```python
from build123d import *

# Parameters (mm, degrees)
BOSS_EXTRUDE1_DEPTH = 90
BOSS_EXTRUDE2_DEPTH = 38


with BuildPart() as part:
    # Sketch1 → Boss-Extrude1 (new body)
    with BuildSketch(Plane.XY):
        with BuildLine():
            Line((-5, -16.770509831), (-5, -12.8))
            Line((-5, -12.8), (5, -12.8))
            Line((5, -12.8), (5, -16.770509831))
            ThreePointArc((5, -16.770509831), (0, 17.5), (-5, -16.770509831))
        make_face()
    extrude(amount=BOSS_EXTRUDE1_DEPTH)

    # Sketch2 → Boss-Extrude2 (add)
    with BuildSketch(Plane(origin=(0, 0, 0), x_dir=(-1, 0, 0), z_dir=(0, 0, -1))):
        with BuildLine():
            ThreePointArc((-5, -16.770509831), (0, -17.5), (5, -16.770509831))
            Line((5, -16.770509831), (5, -12.8))
            Line((5, -12.8), (-5, -12.8))
            Line((-5, -12.8), (-5, -16.770509831))
        make_face()
    extrude(amount=-BOSS_EXTRUDE2_DEPTH)


solid = part.part
```
Read the model definition and answer for the solid it produces. Units are mm, in the model's axes. A direction names the side the tool comes from. Round coordinates to 2 decimals unless told otherwise and drop trailing zeros. Write each loop counter-clockwise with the first axis right and the second up, starting at its lowest first coordinate (ties: lowest second). Pieces come first, ordered by that corner, then holes. Notation, with made-up numbers: (46, 87) - (98, 87) arc R33 ccw to (98, 120) - close; hole circle Ø4 at (15.25, 63.25). An arc over 180 degrees is marked (long way). One line per item, written item: value.
Q1. Each of these flat-tipped pins is pushed along its axis until it touches: P1, Ø10, axis at y = -6.5, z = 39.5, coming from the -X side; P2, Ø11, axis at x = 0.5, z = 56, coming from the -Y side; P3, Ø5, axis at x = 2, z = 47.5, coming from the -Y side. Where does it stop, or does it pass through?
The answers:
P1: stops at x = -17.44
P2: stops at y = -16.77
P3: stops at y = -12.8
Q2. Find section C-C (z = 52). Determine the outline of the cut face in (x, y), and give its area (3 significant figures).
The answers:
outline: (-5, -16.77) - (-5, -12.8) - (5, -12.8) - (5, -16.77) arc R17.5 ccw (long way) to start
area: 918 mm2
Q3. For a pull along X with two mould halves and no side action, classify faces 1 (the flat face through (-5, -15, 64)), 2 (the flat face through (0, 0, 0)) as pulls with the +X half, pulls with the -X half, needs draft (parallel to the pull), parting line crosses it, or undercut.
The answers:
face 1: undercut
face 2: needs draft
Q4. Find section B-B (y = 14). Determine the outline of the cut face in (x, z), and give its area (3 significant figures).
The answers:
outline: (-10.5, 0) - (10.5, 0) - (10.5, 90) - (-10.5, 90) - close
area: 1,890 mm2
Q5. Find section D-D (z = 31). Determine the outline of the cut face in (x, y), and give its area (3 significant figures).
The answers:
outline: circle Ø35 at (0, 0)
area: 962 mm2
Q6. Which of the six approach directions +Z, -Z, +X, -X, +Y, -Y give full straight-line access (tool end or side, diameter ignored) to faces 3 (the flat face through (0, 1, 90)), 4 (the flat face through (5, -15, 64))?
The answers:
face 3: +Z, +X, -X, +Y, -Y
face 4: +Z, -Y
Q7. Find section A-A (x = 0). Determine the outline of the cut face in (y, z), and give its area (3 significant figures).
The answers:
outline: (-17.5, 0) - (17.5, 0) - (17.5, 90) - (-12.8, 90) - (-12.8, 38) - (-17.5, 38) - close
area: 2,910 mm2
Q8. Straight lines are drawn through the part: line 1 (Y direction, x = 0, z = 24); line 2 (Y direction, x = -0.5, z = 78); line 3 (X direction, y = 0.5, z = 30). For each, find the intervals that lie inside material, in ascending order. Write a range as from..to.
The answers:
line 1: y = -17.5..17.5
line 2: y = -12.8..17.49
line 3: x = -17.49..17.49
